```python
from build123d import *

# Parameters (mm, degrees)
BASENUT_START = -5.7404
BASENUTSKE_R  = 2.7051
BASENUT_DEPTH = 5.7404
SCALE1_SCALE  = 0.66


# Read off the part's stored shape, not the designer's step: ThreadSchematic
with BuildPart() as part:
    # BaseNutSke → BaseNut (new body)
    with BuildSketch(Plane.XY.offset(BASENUT_START)):
        Polygon((5.55625, 3.207902433), (5.55625, -3.207902433), (0, -6.415804866), (-5.55625, -3.207902433), (-5.55625, 3.207902433), (0, 6.415804866), align=None)
        Circle(BASENUTSKE_R, mode=Mode.SUBTRACT)
    extrude(amount=BASENUT_DEPTH)

    # Sketch5 (on Front Plane) → EndChamfer (revolve, cut)
    with BuildSketch(Plane.XY):
        Polygon((5.715, 3.175), (5.353069726, 2.65811), (5.7658, 2.65811), (5.7658, 3.175), align=None)
    revolve(axis=Axis((5.715, 3.175, 0), (-0.5735764363510442, -0.8191520442889932, 0)), mode=Mode.SUBTRACT)

    # Sketch3 → Double-Chamfer (revolve, cut)
    with BuildSketch(Plane(origin=(0, 0, 0), x_dir=(0, 0, -1), z_dir=(1, 0, 0))):
        Polygon((5.7404, 5.55625), (5.1054, 6.415804866), (5.1054, 19.115804866), (18.4404, 19.115804866), (18.4404, 5.55625), align=None)
        Polygon((0.635, 19.115804866), (-12.7, 19.115804866), (-12.7, 5.55625), (0, 5.55625), (0.635, 6.415804866), align=None)
    revolve(axis=Axis((0, 0, 0), (0, 0, -1)), mode=Mode.SUBTRACT)

    # ThreadSchematic outline → ThreadSchematic (revolve, cut)
    with BuildSketch(Plane.XZ):
        Polygon((2.7051, 0), (2.7051, -0.329027522), (3.175, 0), align=None)
        Polygon((3.175, -5.715), (2.7051, -5.385972478), (2.7051, -5.7404), (3.175, -5.7404), align=None)
    revolve(axis=Axis((0, 0, 0), (0, 0, 1)), mode=Mode.SUBTRACT)


with BuildPart() as part_1:
    # Scale1: scaled about (0, 0, -2.868948271)
    add(part.part.scale(SCALE1_SCALE).moved(Location((0, 0, -0.975442412))))


solid = part_1.part
```
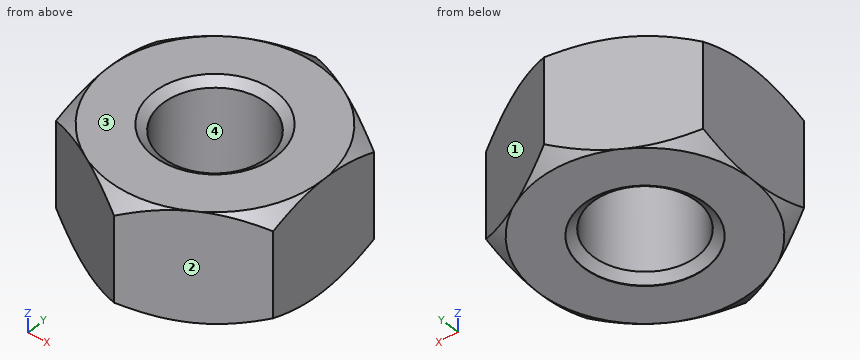
Check sheet for the modelled part. Datum: model origin and axes. Units: mm. Face numbers are marked on the shaded views. Coordinates: 2 decimals unless noted, no trailing zeros. Loops run counter-clockwise (first coordinate to the right, second up) from the corner with the lowest first, then second, coordinate; pieces in that order, holes last.
1) Sectioned sample at A-A (z = -4.1). Record the boundary of the cut face in (x, y).
2) Material ranges on probe 1 along Y at (x, z) = (-1, -4.45); probe 2 along Y at (x, z) = (1.5, -2.95); probe 3 along Z at (x, y) = (1.25, 1.5), recorded low to high.
3) Gauge pin test, flat ends, axial feed: pin 1 (1 mm diameter, centred on y = -3, z = -2, fed in from -X); pin 2 (4 mm diameter, centred on x = 0, y = 0, fed in from +Z); pin 3 (3 mm diameter, centred on x = 0, y = 0, fed in from -Z); pin 4 (1.5 mm diameter, centred on y = 3, z = -2.5, fed in from +X). Record the tip position at first contact, or that the pin passes through.
4) Release check for a two-part mould opening along Y. For the marked faces 1, 2, 3 and 4 record: released by +Y, released by -Y, zero draft, split by the parting line, or undercut.
Check sheet entries:
1. outline: (-3.67, -2.12) - (0, -4.23) - (3.67, -2.12) - (3.67, 2.12) - (0, 4.23) - (-3.67, 2.12) - close; hole circle Ø3.57 at (0, 0)
2. probe 1: y = -3.66 to -1.48, 1.48 to 3.66
2. probe 2: y = -3.37 to -0.97, 0.97 to 3.37
2. probe 3: z = -4.65 to -1.08
3. pin 1: stops at x = -3
3. pin 2: stops at z = -1.04
3. pin 3: passes through
3. pin 4: stops at x = 3.44
4. face 1: released by +Y
4. face 2: released by -Y
4. face 3: zero draft
4. face 4: undercut
